from build123d import *

# Parameters (mm, degrees)
F0_R     = 5
F1_DEPTH = 9.8
F2_W     = 100
F2_H     = 60
F3_DEPTH = 10
F5_DEPTH = 10


with BuildPart() as f1:
    # F0 (on Front) → F1 (new body)
    with BuildSketch(Plane.XZ):
        with BuildLine():
            Line((50, -24.543892), (8.660254, 47.058649))
            ThreePointArc((8.660254, 47.058649), (0, 52.058649), (-8.660254, 47.058649))
            Line((-8.660254, 47.058649), (-50, -24.543892))
            Line((-50, -24.543892), (50, -24.543892))
        make_face()
        with Locations((0, 42.058649)):
            Circle(F0_R, mode=Mode.SUBTRACT)
    extrude(amount=F1_DEPTH)

    # F2 (on face) → F3 (join)
    with BuildSketch(Plane(origin=(0, 0, -24.543892), x_dir=(1, 0, 0), z_dir=(0, 0, -1))):
        with Locations((0, 30)):
            Rectangle(F2_W, F2_H)
    extrude(amount=F3_DEPTH)

    # F4 (on face) → F5 (join)
    with BuildSketch(Plane.XZ.offset(60)):
        Polygon((-35, -14.543892), (-50, -24.543892), (-50, -34.543892), (-30, -34.543892), (-30, -14.543892), align=None)
        Polygon((50, -34.543892), (50, -24.543892), (35, -14.543892), (30, -14.543892), (30, -34.543892), align=None)
    extrude(amount=F5_DEPTH)


solid = f1.part
Input: part model. Units: mm. Frame: model coordinates. A direction names the side the tool comes from. Give positions to 0.01 mm unless a question says otherwise; leave off trailing zeros. Order: outer loops, then holes, each group sorted by start corner. A loop starts at its lowest first (then second) coordinate and runs counter-clockwise, first axis right, second up. Notation, with made-up numbers: M 40.5,85 L 93.5,85 A15 ccw 93.5,102 Z; hole C 16,55.25 d11. An arc over 180 degrees is marked long. Answer as a JSON object with one key per item and string values.
1. Reachability of faces 4 (the flat face through (42.6, -64.93, -19.61)), 5 (the flat face through (0, -60, -29)), 6 (the flat face through (-1, -35, -24.544)), 7 (the flat face through (-32, -65, -14.544)) from +Z, -Z, +X, -X, +Y, -Y: full face, straight path, thin tool, end or side. Return the list, or none.
Result sheet:
{"face 4": "+Z, +X, -Y", "face 5": "+Z, -Z, -Y", "face 6": "+Z, +X, -X", "face 7": "+Z, +X, -X, -Y"}
2. Cut plane A-A, the plane y = -64. Output: boundary loops of the cut face in (x, z).
Result sheet:
{"outline": "M -50,-34.54 L -30,-34.54 L -30,-14.54 L -35,-14.54 L -50,-24.54 Z; M 30,-34.54 L 50,-34.54 L 50,-24.54 L 35,-14.54 L 30,-14.54 Z"}
3. Ray query, line 1 (Z direction, x = -8.5, y = -31); line 2 (Y direction, x = 26.5, z = 6); line 3 (Z direction, x = -34, y = -64). Return the intervals inside material, ascending. Write a range as [from, to].
Result sheet:
{"line 1": "[-34.54, -24.54]", "line 2": "[-9.8, 0]", "line 3": "[-34.54, -14.54]"}
4. First-contact query: P1, Ø3, axis at x = -32.5, z = -9.5, coming from the -Y side; P2, Ø4, axis at x = -1, z = 27.5, coming from the +Y side; P3, Ø3, axis at x = -12, z = -31, coming from the -Y side; P4, Ø25, axis at x = 7, y = -44, coming from the +Z side. Flat tips, straight axial feed; report the tip coordinate or a pass-through.
Result sheet:
{"P1": "y = -9.8", "P2": "y = 0", "P3": "y = -60", "P4": "z = -24.54"}
5. Pull-direction query (Z, two-part tool) for faces 1 (the cylindrical face through (0.147, -4.831, 52.058)), 2 (the flat face through (-30, -65, -25)), 3 (the cylindrical face through (-1.084, -4.831, 37.178)); classes: +Z half, -Z half, draft (parallel to the pull), parting line (faces both ways), or undercut.
Result sheet:
{"face 1": "+Z half", "face 2": "draft", "face 3": "undercut"}
6. Cut plane C-C, the plane y = -5. Output: boundary loops of the cut face in (x, z), and give its area (3 significant figures).
Result sheet:
{"outline": "M -50,-34.54 L 50,-34.54 L 50,-24.54 L 8.66,47.06 A10 ccw -8.66,47.06 L -50,-24.54 Z; hole C 0,42.06 d10", "area": "5,180 mm²"}
7. Cut plane B-B, the plane x = 0. Output: boundary loops of the cut face in (y, z), and give its area (3 significant figures).
Result sheet:
{"outline": "M -60,-34.54 L 0,-34.54 L 0,37.06 L -9.8,37.06 L -9.8,-24.54 L -60,-24.54 Z; M -9.8,47.06 L 0,47.06 L 0,52.06 L -9.8,52.06 Z", "area": "1,250 mm²"}
8. Cut plane D-D, the plane x = 14. Output: boundary loops of the cut face in (y, z).
Result sheet:
{"outline": "M -60,-34.54 L 0,-34.54 L 0,37.81 L -9.8,37.81 L -9.8,-24.54 L -60,-24.54 Z"}
